from build123d import *

# Parameters (mm, degrees)
SKETCH1_W           = 165
SKETCH1_H           = 430
BOSS_EXTRUDE1_DEPTH = 6.25
SKETCH2_W           = 110
SKETCH2_H           = 46
BOSS_EXTRUDE2_DEPTH = 6.25
SKETCH3_R           = 3.15
CUT_EXTRUDE1_DEPTH  = 252.97085645
CUT_EXTRUDE3_DEPTH  = 252.97085645
SKETCH4_W           = 152
SKETCH4_H           = 65
CUT_EXTRUDE2_DEPTH  = 252.97085645
BOSS_EXTRUDE3_DEPTH = 6.25
CUT_EXTRUDE4_DEPTH  = 257.708127063
SKETCH14_W          = 13.5
SKETCH14_H          = 229.5
BOSS_EXTRUDE4_DEPTH = 6.25
FILLET1_R           = 2
SKETCH8_R           = 1.65
CUT_EXTRUDE5_DEPTH  = 257.708127063
CUT_EXTRUDE8_DEPTH  = 257.708127063
LPATTERN1_COUNT     = 3
LPATTERN1_PITCH     = 70
SKETCH9_R           = 2.25
CUT_EXTRUDE6_DEPTH  = 257.708127063
SKETCH10_R          = 1.3
CUT_EXTRUDE7_DEPTH  = 257.708127063
FILLET2_R           = 10
SKETCH13_R          = 3.15
CUT_EXTRUDE9_DEPTH  = 257.708127063
CUT_EXTRUDE10_DEPTH = 257.708127063
FILLET3_R           = 2
SKETCH16_R          = 1.75
CUT_EXTRUDE11_DEPTH = 257.708127063


with BuildPart() as part:
    # Sketch1 → Boss-Extrude1 (new body)
    with BuildSketch(Plane(origin=(0, 0, 0), x_dir=(1, 0, 0), z_dir=(0, 1, 0))):
        Rectangle(SKETCH1_W, SKETCH1_H)
    extrude(amount=BOSS_EXTRUDE1_DEPTH)

    # Sketch2 → Boss-Extrude2 (add)
    with BuildSketch(Plane(origin=(0, 6.25, 0), x_dir=(1, 0, 0), z_dir=(0, 1, 0))):
        with Locations((0, 215)):
            Rectangle(SKETCH2_W, SKETCH2_H)
    extrude(amount=-BOSS_EXTRUDE2_DEPTH)

    # Sketch3 → Cut-Extrude1 (cut, through all)
    with BuildSketch(Plane(origin=(0, 6.25, 0), x_dir=(1, 0, 0), z_dir=(0, 1, 0))):
        with Locations(Location((-45, 228, 0), (0, 0, 270))):
            Circle(SKETCH3_R)
        with Locations(Location((45, 228, 0), (0, 0, 270))):
            Circle(SKETCH3_R)
    extrude(amount=-CUT_EXTRUDE1_DEPTH, mode=Mode.SUBTRACT)

    # Sketch5 → Cut-Extrude3 (cut, through all)
    with BuildSketch(Plane(origin=(0, 6.25, 0), x_dir=(1, 0, 0), z_dir=(0, 1, 0))):
        with BuildLine():
            Line((-78.15, -93.5), (-78.15, -90.5))
            ThreePointArc((-78.15, -90.5), (-75, -87.35), (-71.85, -90.5))
            Line((-71.85, -90.5), (-71.85, -93.5))
            ThreePointArc((-71.85, -93.5), (-75, -96.65), (-78.15, -93.5))
        make_face()
        with BuildLine():
            Line((71.85, -93.5), (71.85, -90.5))
            ThreePointArc((71.85, -90.5), (75, -87.35), (78.15, -90.5))
            Line((78.15, -90.5), (78.15, -93.5))
            ThreePointArc((78.15, -93.5), (75, -96.65), (71.85, -93.5))
        make_face()
    extrude(amount=-CUT_EXTRUDE3_DEPTH, mode=Mode.SUBTRACT)

    # Sketch4 → Cut-Extrude2 (cut, through all)
    with BuildSketch(Plane(origin=(0, 6.25, 0), x_dir=(1, 0, 0), z_dir=(0, 1, 0))):
        with Locations((0, -39.5)):
            Rectangle(SKETCH4_W, SKETCH4_H)
        with Locations((0, -144.5)):
            Rectangle(SKETCH4_W, SKETCH4_H)
    extrude(amount=-CUT_EXTRUDE2_DEPTH, mode=Mode.SUBTRACT)

    # Sketch6 → Boss-Extrude3 (add)
    with BuildSketch(Plane(origin=(0, 6.25, 0), x_dir=(1, 0, 0), z_dir=(0, 1, 0))):
        Polygon((82.5, 0.5), (82.5, -79.5), (96, -64.5), (96, -14.5), align=None)
        Polygon((82.5, -104.5), (82.5, -184.5), (96, -169.5), (96, -119.5), align=None)
    boss_extrude3 = extrude(amount=-BOSS_EXTRUDE3_DEPTH)

    # Sketch7 → Cut-Extrude4 (cut, through all)
    with BuildSketch(Plane(origin=(0, 6.25, 0), x_dir=(1, 0, 0), z_dir=(0, 1, 0))):
        with BuildLine():
            Line((44, -82), (56, -82))
            ThreePointArc((56, -82), (66, -92), (56, -102))
            Line((56, -102), (44, -102))
            ThreePointArc((44, -102), (34, -92), (44, -82))
        make_face()
    cut_extrude4 = extrude(amount=-CUT_EXTRUDE4_DEPTH, mode=Mode.SUBTRACT)

    # Sketch14 → Boss-Extrude4 (add)
    with BuildSketch(Plane(origin=(0, 6.25, 0), x_dir=(1, 0, 0), z_dir=(0, 1, 0))):
        with Locations((89.25, 100.25)):
            Rectangle(SKETCH14_W, SKETCH14_H)
    boss_extrude4 = extrude(amount=-BOSS_EXTRUDE4_DEPTH)

    # Mirror1: Boss-Extrude3, Cut-Extrude4, Boss-Extrude4 across plane
    add(boss_extrude3.mirror(Plane(origin=(0, 0, 0), x_dir=(0, 0, 1), z_dir=(1, 0, 0))))
    add(cut_extrude4.mirror(Plane(origin=(0, 0, 0), x_dir=(0, 0, 1), z_dir=(1, 0, 0))), mode=Mode.SUBTRACT)
    add(boss_extrude4.mirror(Plane(origin=(0, 0, 0), x_dir=(0, 0, 1), z_dir=(1, 0, 0))))

    # Fillet1
    fillet1_edges = [part.edges().sort_by_distance(p)[0] for p in [
        (76, 3.125, 7),
        (76, 3.125, 72),
        (-76, 3.125, 72),
        (-76, 3.125, 7),
        (76, 3.125, 112),
        (76, 3.125, 177),
        (-76, 3.125, 177),
        (-76, 3.125, 112),
    ]]
    fillet(fillet1_edges, radius=FILLET1_R)

    # Sketch8 → Cut-Extrude5 (cut, through all)
    with BuildSketch(Plane(origin=(0, 6.25, 0), x_dir=(1, 0, 0), z_dir=(0, 1, 0))):
        with Locations(Location((39, 207, 0), (0, 0, 270))):
            Circle(SKETCH8_R)
        with Locations(Location((88, 207, 0), (0, 0, 270))):
            Circle(SKETCH8_R)
        with Locations(Location((88, 158, 0), (0, 0, 270))):
            Circle(SKETCH8_R)
        with Locations(Location((39, 158, 0), (0, 0, 270))):
            Circle(SKETCH8_R)
    cut_extrude5 = extrude(amount=-CUT_EXTRUDE5_DEPTH, mode=Mode.SUBTRACT)

    # Sketch12 → Cut-Extrude8 (cut, through all)
    with BuildSketch(Plane(origin=(0, 6.25, 0), x_dir=(1, 0, 0), z_dir=(0, 1, 0))):
        with BuildLine():
            Line((28, 172.5), (28, 192.5))
            ThreePointArc((28, 192.5), (31, 195.5), (34, 192.5))
            Line((34, 192.5), (34, 172.5))
            ThreePointArc((34, 172.5), (31, 169.5), (28, 172.5))
        make_face()
    cut_extrude8 = extrude(amount=-CUT_EXTRUDE8_DEPTH, mode=Mode.SUBTRACT)

    # LPattern1: Cut-Extrude5, Cut-Extrude8 ×3
    with Locations(*[(0, 0, i * LPATTERN1_PITCH) for i in range(1, LPATTERN1_COUNT)]):
        add(cut_extrude5, mode=Mode.SUBTRACT)
        add(cut_extrude8, mode=Mode.SUBTRACT)

    # Sketch9 → Cut-Extrude6 (cut, through all)
    with BuildSketch(Plane(origin=(0, 6.25, 0), x_dir=(1, 0, 0), z_dir=(0, 1, 0))):
        with Locations(Location((-88, 86, 0), (0, 0, 270))):
            Circle(SKETCH9_R)
        with Locations(Location((-18, 86, 0), (0, 0, 270))):
            Circle(SKETCH9_R)
        with Locations(Location((-88, 13, 0), (0, 0, 270))):
            Circle(SKETCH9_R)
        with Locations(Location((-18, 13, 0), (0, 0, 270))):
            Circle(SKETCH9_R)
    extrude(amount=-CUT_EXTRUDE6_DEPTH, mode=Mode.SUBTRACT)

    # Sketch10 → Cut-Extrude7 (cut, through all)
    with BuildSketch(Plane(origin=(0, 6.25, 0), x_dir=(1, 0, 0), z_dir=(0, 1, 0))):
        with Locations(Location((-88, 200, 0), (0, 0, 270))):
            Circle(SKETCH10_R)
        with Locations(Location((-30, 200, 0), (0, 0, 270))):
            Circle(SKETCH10_R)
        with Locations(Location((-88, 151, 0), (0, 0, 270))):
            Circle(SKETCH10_R)
        with Locations(Location((-30, 151, 0), (0, 0, 270))):
            Circle(SKETCH10_R)
    extrude(amount=-CUT_EXTRUDE7_DEPTH, mode=Mode.SUBTRACT)

    # Fillet2
    fillet2_edges = [part.edges().sort_by_distance(p)[0] for p in [
        (82.5, 3.125, 79.5),
        (82.5, 3.125, 104.5),
        (-82.5, 3.125, 79.5),
        (-82.5, 3.125, 104.5),
    ]]
    fillet(fillet2_edges, radius=FILLET2_R)

    # Sketch13 → Cut-Extrude9 (cut, through all)
    with BuildSketch(Plane(origin=(0, 6.25, 0), x_dir=(1, 0, 0), z_dir=(0, 1, 0))):
        with Locations(Location((-70, -205, 0), (0, 0, 270))):
            Circle(SKETCH13_R)
        with Locations(Location((70, -205, 0), (0, 0, 270))):
            Circle(SKETCH13_R)
        with Locations(Location((0, -205, 0), (0, 0, 270))):
            Circle(SKETCH13_R)
    extrude(amount=-CUT_EXTRUDE9_DEPTH, mode=Mode.SUBTRACT)

    # Sketch15 → Cut-Extrude10 (cut, through all)
    with BuildSketch(Plane(origin=(0, 6.25, 0), x_dir=(1, 0, 0), z_dir=(0, 1, 0))):
        with BuildLine():
            Line((-88, 122.65), (-86, 122.65))
            ThreePointArc((-86, 122.65), (-84.35, 121), (-86, 119.35))
            Line((-86, 119.35), (-88, 119.35))
            ThreePointArc((-88, 119.35), (-89.65, 121), (-88, 122.65))
        make_face()
        with BuildLine():
            Line((20, 119.35), (18, 119.35))
            ThreePointArc((18, 119.35), (16.35, 121), (18, 122.65))
            Line((18, 122.65), (20, 122.65))
            ThreePointArc((20, 122.65), (21.65, 121), (20, 119.35))
        make_face()
    extrude(amount=-CUT_EXTRUDE10_DEPTH, mode=Mode.SUBTRACT)

    # Fillet3
    fillet3_edges = [part.edges().sort_by_distance(p)[0] for p in [
        (96, 3.125, 64.5),
        (82.5, 3.125, 184.5),
        (96, 3.125, 169.5),
        (96, 3.125, 119.5),
        (96, 3.125, -215),
        (-96, 3.125, 64.5),
        (-96, 3.125, 119.5),
        (-82.5, 3.125, 184.5),
        (-96, 3.125, 169.5),
        (55, 3.125, -238),
        (-96, 3.125, -215),
        (-55, 3.125, -238),
        (-55, 3.125, -215),
        (55, 3.125, -215),
        (82.5, 3.125, 215),
        (-82.5, 3.125, 215),
    ]]
    fillet(fillet3_edges, radius=FILLET3_R)

    # Sketch16 → Cut-Extrude11 (cut, through all)
    with BuildSketch(Plane(origin=(0, 6.25, 0), x_dir=(1, 0, 0), z_dir=(0, 1, 0))):
        with Locations(Location((-25, 211, 0), (0, 0, 270))):
            Circle(SKETCH16_R)
        with Locations(Location((32, 211, 0), (0, 0, 270))):
            Circle(SKETCH16_R)
    extrude(amount=-CUT_EXTRUDE11_DEPTH, mode=Mode.SUBTRACT)


solid = part.part
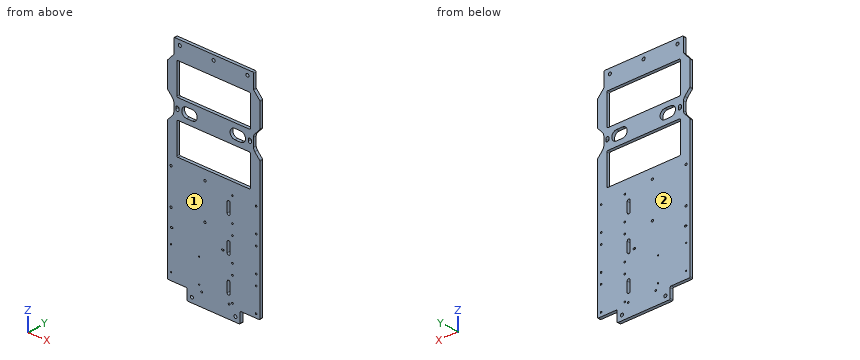
For this review, take the finished solid that the model builds, in its own axes (mm). Face numbers are marked on the shaded views. Round coordinates to 2 decimals unless told otherwise and drop trailing zeros. Use a Markdown table: item, result.
Q1. Wall thickness on line 1 along Z through (x, y) = (14.5, 5.75); line 2 along X through (y, z) = (5, -211); line 3 along X through (y, z) = (1.5, -207): over which ranges is each line inside the solid? List them lowest first.
Derived:
| item | result |
|---|---|
| line 1 | z = -238 to 7, 72 to 112, 177 to 215 |
| line 2 | x = -96 to -26.75, -23.25 to 30.25, 33.75 to 96 |
| line 3 | x = -96 to 37.35, 40.65 to 86.35, 89.65 to 96 |
Q2. Clearance check with flat-ended pins moving along their axes: pin 1 (1 mm diameter, centred on y = 4.5, z = 97.5, fed in from -X); pin 2 (12 mm diameter, centred on x = -68.5, z = -104.5, fed in from -Y); pin 3 (3.5 mm diameter, centred on y = 3, z = 92.5, fed in from +X). State where each tip first meets the part, or that it passes through.
Derived:
| item | result |
|---|---|
| pin 1 | stops at x = -82.5 |
| pin 2 | stops at y = 0 |
| pin 3 | stops at x = 82.5 |
Q3. We need section A-A (y = 1). State how many separate pieces and enclosed holes the cut face has, plus the area to 3 significant figures.
Derived:
| item | result |
|---|---|
| separate pieces | 1 |
| enclosed holes | 38 |
| area | 61,200 mm2 |
Q4. The part is to be moulded in two halves that separate along Y. For the marked faces 1 and 2, say which applies: pulls with the +Y half, pulls with the -Y half, needs draft (parallel to the pull), parting line crosses it, or undercut.
Derived:
| item | result |
|---|---|
| face 1 | pulls with the -Y half |
| face 2 | pulls with the +Y half |
